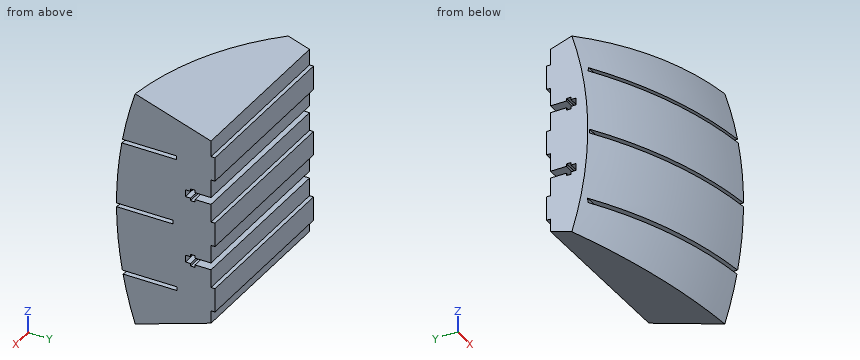
from build123d import *

# Parameters (mm, degrees)
REVOLVE1_ANGLE      = 36
SKETCH2_W           = 185.252199215
SKETCH2_H           = 56.371609172
CUT_EXTRUDE1_DEPTH  = 365.059347887
SKETCH5_W           = 55.655123519
SKETCH5_H           = 148.553285118
CUT_EXTRUDE2_DEPTH  = 235.735844279
SKETCH6_W           = 162.024812579
SKETCH6_H           = 19.05
BOSS_EXTRUDE1_DEPTH = 3.175
LPATTERN1_COUNT     = 3
LPATTERN1_PITCH     = 53.34
CUT_EXTRUDE3_DEPTH  = 357.818950588
LPATTERN2_COUNT     = 2
LPATTERN2_PITCH     = 53.34
SKETCH8_W           = 53.705765401
SKETCH8_H           = 196.003453697
CUT_EXTRUDE4_DEPTH  = 224.765760383
SKETCH10_W          = 3.048
SKETCH10_H          = 86.618344978
SKETCH10_H_2        = 89.651067892
CUT_EXTRUDE6_DEPTH  = 176.53


with BuildPart() as part:
    # Sketch1 → Revolve1 (revolve, symmetric)
    with BuildSketch(Plane.XY) as revolve1_sk:
        with BuildLine():
            Line((-202.80204389, -227.539822875), (-25.4, -227.539822875))
            Line((-25.4, -227.539822875), (-25.4, -303.739822875))
            ThreePointArc((-25.4, -303.739822875), (-120.294028152, -280.057827584), (-202.80204389, -227.539822875))
        make_face()
    revolve(axis=Axis((0, 0, 0), (-1, 0, 0)), revolution_arc=REVOLVE1_ANGLE / 2)
    revolve(revolve1_sk.sketch, axis=Axis((0, 0, 0), (1, 0, 0)), revolution_arc=REVOLVE1_ANGLE / 2)

    # Sketch2 → Cut-Extrude1 (cut, through all)
    with BuildSketch(Plane(origin=(-25.4, 0, 0), x_dir=(0, 0, -1), z_dir=(1, 0, 0))):
        with Locations((3.182919918, -200.414195414)):
            Rectangle(SKETCH2_W, SKETCH2_H)
    extrude(amount=-CUT_EXTRUDE1_DEPTH, mode=Mode.SUBTRACT)

    # Sketch5 → Cut-Extrude2 (cut, through all)
    with BuildSketch(Plane(origin=(0, -228.6, 0), x_dir=(1, 0, 0), z_dir=(0, 1, 0))):
        with Locations((-215.252374339, 0)):
            Rectangle(SKETCH5_W, SKETCH5_H)
    extrude(amount=-CUT_EXTRUDE2_DEPTH, mode=Mode.SUBTRACT)

    # Sketch6 → Boss-Extrude1 (add)
    with BuildSketch(Plane(origin=(0, -228.6, 0), x_dir=(1, 0, 0), z_dir=(0, 1, 0))):
        with Locations((-106.41240629, -52.051642559)):
            Rectangle(SKETCH6_W, SKETCH6_H)
    boss_extrude1 = extrude(amount=BOSS_EXTRUDE1_DEPTH)

    # LPattern1: Boss-Extrude1 ×3
    with Locations(*[(0, 0, -i * LPATTERN1_PITCH) for i in range(1, LPATTERN1_COUNT)]):
        add(boss_extrude1)

    # Sketch7 → Cut-Extrude3 (cut, through all)
    with BuildSketch(Plane(origin=(-25.4, 0, 0), x_dir=(0, 0, -1), z_dir=(1, 0, 0))):
        with BuildLine():
            Line((-22.603517559, -244.856), (-22.603517559, -248.92))
            Line((-22.603517559, -248.92), (-28.159767559, -248.92))
            Line((-28.159767559, -248.92), (-28.159767559, -244.856))
            Line((-28.159767559, -244.856), (-30.144142559, -244.856))
            Line((-30.144142559, -244.856), (-30.144142559, -241.427))
            ThreePointArc((-30.144142559, -241.427), (-30.23394512, -241.210197439), (-30.017142559, -241.3))
            Line((-30.017142559, -241.3), (-28.159767559, -241.3))
            Line((-28.159767559, -241.3), (-28.159767559, -228.6))
            Line((-28.159767559, -228.6), (-22.603517559, -228.6))
            Line((-22.603517559, -228.6), (-22.603517559, -241.3))
            Line((-22.603517559, -241.3), (-20.746142559, -241.3))
            ThreePointArc((-20.746142559, -241.3), (-20.529339998, -241.210197439), (-20.619142559, -241.427))
            Line((-20.619142559, -241.427), (-20.619142559, -244.856))
            Line((-20.619142559, -244.856), (-22.603517559, -244.856))
        make_face()
    cut_extrude3 = extrude(amount=-CUT_EXTRUDE3_DEPTH, mode=Mode.SUBTRACT)

    # LPattern2: Cut-Extrude3 ×2
    with Locations(*[(0, 0, -i * LPATTERN2_PITCH) for i in range(1, LPATTERN2_COUNT)]):
        add(cut_extrude3, mode=Mode.SUBTRACT)

    # Sketch8 → Cut-Extrude4 (cut, through all)
    with BuildSketch(Plane(origin=(0, -225.425, 0), x_dir=(1, 0, 0), z_dir=(0, 1, 0))):
        with Locations((-188.777882701, -12.617417505)):
            Rectangle(SKETCH8_W, SKETCH8_H)
    extrude(amount=-CUT_EXTRUDE4_DEPTH, mode=Mode.SUBTRACT)

    # Sketch10 → Cut-Extrude6 (cut)
    with BuildSketch(Plane(origin=(0, 0, 0), x_dir=(0, 0, -1), z_dir=(1, 0, 0))):
        with Locations((54.628357441, -298.786918327)):
            Rectangle(SKETCH10_W, SKETCH10_H)
        with Locations((1.288357441, -303.737090483)):
            Rectangle(SKETCH10_W, SKETCH10_H_2)
        with Locations((-52.051642559, -299.246564737)):
            Rectangle(SKETCH10_W, SKETCH10_H)
    extrude(amount=-CUT_EXTRUDE6_DEPTH, mode=Mode.SUBTRACT)


solid = part.part
Verification items for the finished model (mm, model axes). Coordinates: 2 decimals unless noted, no trailing zeros. Order: outer loops, then holes, each group sorted by start corner. A loop starts at its lowest first (then second) coordinate and runs counter-clockwise, first axis right, second up. Notation, with made-up numbers: M -15,-23.75 L 23,-23.75 A20 cw 23,14.25 Z; hole C 21.5,76 d8. An arc over 180 degrees is marked long. One line per item, written item: value. Start each with the question number.
Item 1: Gauge pin test, flat ends, axial feed: pin 1 (8 mm diameter, centred on x = -57.5, y = -255.5, fed in from -Z); pin 2 (1.5 mm diameter, centred on x = -68, z = 22, fed in from -Y); pin 3 (0.6 mm diameter, centred on x = -93.5, z = -24, fed in from -Y). Record the tip position at first contact, or that the pin passes through.
Item 2: Sectioned sample at B-B (z = 3). Enter the section's corners in (x, y) (3 decimals).
Item 3: Sectioned sample at A-A (y = -261). Enter the section's corners in (x, z).
Item 4: Scan lines: probe 1 along Z at (x, y) = (-83, -241); probe 2 along Z at (x, y) = (-97.5, -266); probe 3 along Z at (x, y) = (-58.5, -240). Record each from-to range of solid material in increasing order.
Conclusion:
1. pin 1: stops at z = -84.32
1. pin 2: stops at y = -296.48
1. pin 3: stops at y = -289.21
2. outline: M -161.925,-258.214 A304.785 ccw -25.4,-303.725 L -25.4,-225.425 L -161.925,-225.425 Z
3. outline: M -157.42,0.24 L -25.4,0.24 L -25.4,50.53 L -149.09,50.53 A157.42 ccw Z; M -157.4,-2.81 A157.42 ccw -148.2,-53.1 L -25.4,-53.1 L -25.4,-2.81 Z; M -148.03,53.58 L -25.4,53.58 L -25.4,84.8 L -132.63,84.8 A157.42 ccw Z; M -147.07,-56.15 A157.42 ccw -132.63,-84.8 L -25.4,-84.8 L -25.4,-56.15 Z
4. probe 1: z = -78.31 to -30.74, -25.18 to 22.6, 28.16 to 78.31
4. probe 2: z = -86.43 to -56.15, -53.1 to -2.81, 0.24 to 50.53, 53.58 to 86.43
4. probe 3: z = -77.98 to -30.74, -25.18 to 22.6, 28.16 to 77.98
